```python
from build123d import *

# Parameters (mm, degrees)
SKETCH_1_R          = 1.35
EXTRUDE_1_DEPTH     = 7
FILLET_1_R          = 1
FILLET_2_R          = 1
FILLET_3_R          = 1
FILLET_4_R          = 1
FILLET_5_R          = 10
SKETCH_2_R          = 4
CUT_EXTRUDE_1_DEPTH = 4
SKETCH_3_R          = 6.1
CUT_EXTRUDE_2_DEPTH = 4
SKETCH_4_R          = 7.1
CUT_EXTRUDE_4_DEPTH = 1.6
SKETCH_5_R          = 7.1
CUT_EXTRUDE_5_DEPTH = 1.6
SKETCH_6_R          = 2.25
SKETCH_6_R_2        = 3.5
CUT_EXTRUDE_6_DEPTH = 5
CHAMFER_1_SIZE      = 0.6
CHAMFER_2_SIZE      = 0.5
SKETCH_7_R          = 2.75
CUT_EXTRUDE_7_DEPTH = 2.8


with BuildPart() as part:
    # 草图1 → 凸台-拉伸1 (new body)
    with BuildSketch(Plane(origin=(0, 0, 0), x_dir=(1, 0, 0), z_dir=(0, 1, 0))):
        with BuildLine():
            Line((-120, 10), (-11.180339887, 10))
            ThreePointArc((-11.180339887, 10), (15, 0), (-11.180339887, -10))
            Line((-11.180339887, -10), (-120, -10))
            ThreePointArc((-120, -10), (-130, 0), (-120, 10))
        make_face()
        with Locations(Location((-11, 0, 0), (0, 0, 270))):
            Circle(SKETCH_1_R, mode=Mode.SUBTRACT)
        with Locations(Location((0, 11, 0), (0, 0, 270))):
            Circle(SKETCH_1_R, mode=Mode.SUBTRACT)
        with Locations(Location((11, 0, 0), (0, 0, 270))):
            Circle(SKETCH_1_R, mode=Mode.SUBTRACT)
        with Locations(Location((0, -11, 0), (0, 0, 270))):
            Circle(SKETCH_1_R, mode=Mode.SUBTRACT)
        Polygon((-104.558275962, -5), (-53.32280907, -5), (-78.940542516, 2.906902245), align=None, mode=Mode.SUBTRACT)
        with BuildLine():
            Line((-111.339745962, 5), (-85.722012516, 5))
            Line((-85.722012516, 5), (-110.343778499, -2.599497322))
            ThreePointArc((-110.343778499, -2.599497322), (-110.084789012, 1.299457992), (-111.339745962, 5))
        make_face(mode=Mode.SUBTRACT)
        Polygon((-72.159072516, 5), (-46.54133907, -2.906902245), (-20.923605624, 5), align=None, mode=Mode.SUBTRACT)
        with BuildLine():
            Line((-39.75986907, -5), (-14.751545054, 2.71880829))
            ThreePointArc((-14.751545054, 2.71880829), (-14.953467696, -1.180594709), (-14.142135624, -5))
            Line((-14.142135624, -5), (-39.75986907, -5))
        make_face(mode=Mode.SUBTRACT)
    extrude(amount=EXTRUDE_1_DEPTH)

    # 圆角1
    fillet_1_edges = [part.edges().sort_by_distance(p)[0] for p in [
        (-85.722012516, 3.5, -5),
        (-111.339745962, 3.5, -5),
        (-110.343778499, 3.5, 2.599497322),
    ]]
    fillet(fillet_1_edges, radius=FILLET_1_R)

    # 圆角2
    fillet_2_edges = [part.edges().sort_by_distance(p)[0] for p in [
        (-104.558275962, 3.5, 5),
        (-53.32280907, 3.5, 5),
        (-78.940542516, 3.5, -2.906902245),
    ]]
    fillet(fillet_2_edges, radius=FILLET_2_R)

    # 圆角3
    fillet_3_edges = [part.edges().sort_by_distance(p)[0] for p in [
        (-46.54133907, 3.5, 2.906902245),
        (-20.923605624, 3.5, -5),
        (-72.159072516, 3.5, -5),
    ]]
    fillet(fillet_3_edges, radius=FILLET_3_R)

    # 圆角4
    fillet_4_edges = [part.edges().sort_by_distance(p)[0] for p in [
        (-39.75986907, 3.5, 5),
        (-14.142135624, 3.5, 5),
        (-14.751545054, 3.5, -2.71880829),
    ]]
    fillet(fillet_4_edges, radius=FILLET_4_R)

    # 圆角5
    fillet_5_edges = [part.edges().sort_by_distance(p)[0] for p in [
        (-11.180339887, 3.5, -10),
        (-11.180339887, 3.5, 10),
    ]]
    fillet(fillet_5_edges, radius=FILLET_5_R)

    # 草图2 → 切除-拉伸1 (cut)
    with BuildSketch(Plane(origin=(0, 0, 0), x_dir=(-1, 0, 0), z_dir=(0, -1, 0))):
        with Locations(Location((0, 0, 0), (0, 0, 90))):
            Circle(SKETCH_2_R)
    extrude(amount=-CUT_EXTRUDE_1_DEPTH, mode=Mode.SUBTRACT)

    # 草图3 → 切除-拉伸2 (cut)
    with BuildSketch(Plane(origin=(0, 0, 0), x_dir=(-1, 0, 0), z_dir=(0, -1, 0))):
        with Locations(Location((120, 0, 0), (0, 0, 90))):
            Circle(SKETCH_3_R)
    extrude(amount=-CUT_EXTRUDE_2_DEPTH, mode=Mode.SUBTRACT)

    # 草图4 → 切除-拉伸4 (cut)
    with BuildSketch(Plane(origin=(0, 7, 0), x_dir=(1, 0, 0), z_dir=(0, 1, 0))):
        with Locations(Location((0, 0, 0), (0, 0, 270))):
            Circle(SKETCH_4_R)
    extrude(amount=-CUT_EXTRUDE_4_DEPTH, mode=Mode.SUBTRACT)

    # 草图5 → 切除-拉伸5 (cut)
    with BuildSketch(Plane(origin=(0, 7, 0), x_dir=(1, 0, 0), z_dir=(0, 1, 0))):
        with Locations(Location((-120, 0, 0), (0, 0, 270))):
            Circle(SKETCH_5_R)
    extrude(amount=-CUT_EXTRUDE_5_DEPTH, mode=Mode.SUBTRACT)

    # 草图6 → 切除-拉伸6 (cut, symmetric)
    with BuildSketch(Plane(origin=(0, 5.4, 0), x_dir=(1, 0, 0), z_dir=(0, 1, 0))):
        with Locations(Location((0, 0, 0), (0, 0, 270))):
            Circle(SKETCH_6_R)
        with Locations(Location((-120, 0, 0), (0, 0, 270))):
            Circle(SKETCH_6_R_2)
    extrude(amount=CUT_EXTRUDE_6_DEPTH, both=True, mode=Mode.SUBTRACT)

    # 倒角1
    chamfer_1_edges = [part.edges().sort_by_distance(p)[0] for p in [
        (15, 0, 0),
        (15, 7, 0),
        (-11.83772234, 0, 10.513167019),
        (-11.83772234, 7, 10.513167019),
        (-11.83772234, 0, -10.513167019),
        (-11.83772234, 7, -10.513167019),
        (-130, 0, 0),
        (-67.5, 0, -10),
        (-67.5, 0, 10),
        (-67.5, 7, 10),
        (-67.5, 7, -10),
        (-130, 7, 0),
    ]]
    chamfer(chamfer_1_edges, length=CHAMFER_1_SIZE)

    # 倒角2
    chamfer_2_edges = [part.edges().sort_by_distance(p)[0] for p in [
        (-120, 0, 6.1),
    ]]
    chamfer(chamfer_2_edges, length=CHAMFER_2_SIZE)

    # 草图7 → 切除-拉伸7 (cut)
    with BuildSketch(Plane(origin=(0, 7, 0), x_dir=(1, 0, 0), z_dir=(0, 1, 0))):
        with Locations(Location((0, 11, 0), (0, 0, 270))):
            Circle(SKETCH_7_R)
        with Locations(Location((11, 0, 0), (0, 0, 270))):
            Circle(SKETCH_7_R)
        with Locations(Location((0, -11, 0), (0, 0, 270))):
            Circle(SKETCH_7_R)
        with Locations(Location((-11, 0, 0), (0, 0, 270))):
            Circle(SKETCH_7_R)
    extrude(amount=-CUT_EXTRUDE_7_DEPTH, mode=Mode.SUBTRACT)


solid = part.part
```
Could you check a few things on this model? Use its own coordinates, in mm. A direction names the side the tool comes from. Coordinates: 2 decimals unless noted, no trailing zeros. Write each loop counter-clockwise with the first axis right and the second up, starting at its lowest first coordinate (ties: lowest second). Pieces come first, ordered by that corner, then holes. Notation, with made-up numbers: M 48,58 L 88,58 A8 ccw 88,69 Z; hole C 15.5,65 d11. An arc over 180 degrees is marked long. Answer as CSV lines item,"result". Start each with the question number.
1) We'd pull the mould along X, two halves only. Please class faces 1 (the cylindrical face through (-110.084, 3.451, -1.297)), 2 (the conical face through (-129.6, 0.2, 0.2)), 3 (the flat face through (-41, 7, 3)): +X half, -X half, draft (parallel to the pull), parting line (faces both ways), or undercut.
2) I want a section at B-B, the plane x = -74.5. Please give me the cut outline in (y, z), and give its area (3 significant figures).
3) Please list where these lines run through material, in increasing order: line 1 (Z direction, x = -59.5, y = 4.5); line 2 (X direction, y = 2, z = -11.25); line 3 (Z direction, x = -52, y = 2.5). Write a range as from..to.
4) For P1, Ø3, axis at x = -61.5, y = 6, coming from the -Z side; P2, Ø5, axis at x = 0, z = 0, coming from the -Y side; P3, Ø3.5, axis at x = -99.5, y = 3.5, coming from the +Z side, each with a flat end and sliding along its axis, tell me the tip position at first contact or that it passes through.
5) I want a section at A-A, the plane x = 0. Give the number of separate pieces and of enclosed holes in the cut face, and give its area (3 significant figures).
6) For faces 4 (the flat face through (-88.596, 3.451, 0.073)), 5 (the flat face through (-2, 4, -2)), 6 (the cylindrical face through (-126.93, 6.21, -1.54)), which set-ups out of +Z, -Z, +X, -X, +Y, -Y let a thin tool reach every point of the face, with its end or its side?
Data:
1,face 1,"undercut"
1,face 2,"-X half"
1,face 3,"draft"
2,outline,"M 0,-9.4 L 0.6,-10 L 6.4,-10 L 7,-9.4 L 7,-1.54 L 0,-1.54 Z; M 0,5 L 7,5 L 7,9.4 L 6.4,10 L 0.6,10 L 0,9.4 Z"
2,area,"93.5 mm^2"
3,line 1,"z = -10..-5, -1.09..3.11, 4.89..10"
3,line 2,"x = -10.16..-1.33, 1.33..9.92"
3,line 3,"z = -10..-5, 1.22..10"
4,P1,"stops at z = -10"
4,P2,"stops at y = 4"
4,P3,"stops at z = 10"
5,separate pieces,"4"
5,enclosed holes,"0"
5,area,"94.8 mm^2"
6,face 4,"+Y, -Y"
6,face 5,"-Y"
6,face 6,"+Y"
